Source: CAD feature listing. Evaluate the final solid. Frame: model axes, mm. Face numbers are marked on the shaded views. A direction names the side the tool comes from. Coordinates: 2 decimals unless noted, no trailing zeros. Loops run counter-clockwise (first coordinate to the right, second up) from the corner with the lowest first, then second, coordinate; pieces in that order, holes last.
Item 1: Section query B-B, the plane x = 15.5. Return the cut outline in (y, z), then the cut area to 3 significant figures.
Item 2: Reachability of the marked faces 1, 2, 3 and 4 from +Z, -Z, +X, -X, +Y, -Y: full face, straight path, thin tool, end or side. Return the list, or none.
Item 3: Section query A-A, the plane y = 5.5. Return the cut outline in (x, z), then the cut area to 3 significant figures.
Item 4: Section query C-C, the plane z = 4.5. Return the cut outline in (x, y).
Item 5: Pull-direction query (X, two-part tool) for the marked faces 5, 6, 7 and 8; classes: +X half, -X half, draft (parallel to the pull), parting line (faces both ways), or undercut.
Item 6: Section query D-D, the plane y = 2.5. Return the cut outline in (x, z), then the cut area to 3 significant figures.
Item 7: Pin query (flat end, axial travel): pin 1 Ø0.9 at (y, z) = (9, 0.5) entering from +X; pin 2 Ø1.5 at (y, z) = (6, -2) entering from -X; pin 3 Ø2.5 at (x, y) = (-8, 5.5) entering from +Z; pin 4 Ø3 at (y, z) = (5, -1.5) entering from -X. Return the tip coordinate at first contact, or that it passes through.
Item 8: Line query: probe 1 along Z at (x, y) = (-4, 10); probe 2 along X at (y, z) = (7.5, -0.25); probe 3 along Z at (x, y) = (9.5, 4.5). Output: solid intervals per line, ascending.
```python
from build123d import *

# Parameters (mm, degrees)
SKETCH1_W           = 13.5
SKETCH1_H           = 6.2
BOSS_EXTRUDE1_DEPTH = 11
SKETCH2_R           = 1.6
CUT_EXTRUDE1_DEPTH  = 30.829725108
FILLET1_R           = 1
SKETCH3_W           = 18
SKETCH3_H           = 3
CUT_EXTRUDE2_DEPTH  = 30.829725108


with BuildPart() as part:
    # Sketch1 → Boss-Extrude1 (new body)
    with BuildSketch(Plane(origin=(0, 0, 0), x_dir=(1, 0, 0), z_dir=(0, 1, 0))):
        with BuildLine():
            Line((-12, -6.25), (24.75, -6.25))
            Line((24.75, -6.25), (24.75, 6.25))
            Line((24.75, 6.25), (-12, 6.25))
            Line((-12, 6.25), (-12, 3.5))
            Line((-12, 3.5), (-2.037768387, 3.5))
            ThreePointArc((-2.037768387, 3.5), (2.018605711, 3.511086867), (4.05, 0))
            ThreePointArc((4.05, 0), (2.018605711, -3.511086867), (-2.037768387, -3.5))
            Line((-2.037768387, -3.5), (-12, -3.5))
            Line((-12, -3.5), (-12, -6.25))
        make_face()
        with Locations((15, 0)):
            Rectangle(SKETCH1_W, SKETCH1_H, mode=Mode.SUBTRACT)
    extrude(amount=BOSS_EXTRUDE1_DEPTH)

    # Sketch2 → Cut-Extrude1 (cut, through all)
    with BuildSketch(Plane.XY.offset(6.25)):
        with Locations((-8, 5.5)):
            Circle(SKETCH2_R)
    extrude(amount=-CUT_EXTRUDE1_DEPTH, mode=Mode.SUBTRACT)

    # Fillet1
    fillet1_edges = [part.edges().sort_by_distance(p)[0] for p in [
        (-12, 5.5, -6.25),
        (24.75, 5.5, -6.25),
        (24.75, 5.5, 6.25),
        (-12, 5.5, 6.25),
    ]]
    fillet(fillet1_edges, radius=FILLET1_R)

    # Sketch3 → Cut-Extrude2 (cut, through all)
    with BuildSketch(Plane.XY.offset(6.25)):
        with Locations((15.75, 9.5)):
            Rectangle(SKETCH3_W, SKETCH3_H)
    extrude(amount=-CUT_EXTRUDE2_DEPTH, mode=Mode.SUBTRACT)


solid = part.part
```
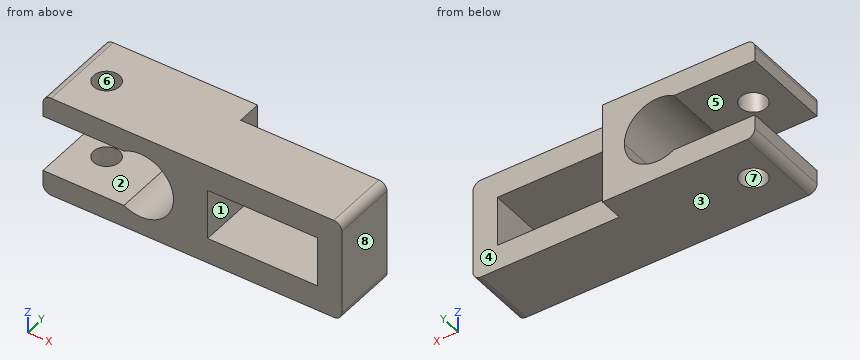
Verdict:
1. outline: (0, -6.25) - (8, -6.25) - (8, -3.1) - (0, -3.1) - close; (0, 3.1) - (8, 3.1) - (8, 6.25) - (0, 6.25) - close
1. area: 50.4 mm2
2. face 1: +Y, -Y
2. face 2: -X, +Y, -Y
2. face 3: -Z, +X, -X, +Y, -Y
2. face 4: +Z, -Z, +X, +Y
3. outline: (-12, -5.25) arc R1 ccw to (-11, -6.25) - (-9.6, -6.25) - (-9.6, -3.5) - (-12, -3.5) - close; (-12, 3.5) - (-9.6, 3.5) - (-9.6, 6.25) - (-11, 6.25) arc R1 ccw to (-12, 5.25) - close; (-6.4, -6.25) - (23.75, -6.25) arc R1 ccw to (24.75, -5.25) - (24.75, 5.25) arc R1 ccw to (23.75, 6.25) - (-6.4, 6.25) - (-6.4, 3.5) - (-2.04, 3.5) arc R4.05 cw (long way) to (-2.04, -3.5) - (-6.4, -3.5) - close; hole (8.25, -3.1) - (21.75, -3.1) - (21.75, 3.1) - (8.25, 3.1) - close
3. area: 246 mm2
4. outline: (-12, 0) - (24.75, 0) - (24.75, 8) - (6.75, 8) - (6.75, 11) - (-12, 11) - close; hole circle Ø3.2 at (-8, 5.5)
5. face 5: draft
5. face 6: undercut
5. face 7: undercut
5. face 8: +X half
6. outline: (-12, -5.25) arc R1 ccw to (-11, -6.25) - (23.75, -6.25) arc R1 ccw to (24.75, -5.25) - (24.75, 5.25) arc R1 ccw to (23.75, 6.25) - (-11, 6.25) arc R1 ccw to (-12, 5.25) - (-12, 3.5) - (-2.04, 3.5) arc R4.05 cw (long way) to (-2.04, -3.5) - (-12, -3.5) - close; hole (8.25, -3.1) - (21.75, -3.1) - (21.75, 3.1) - (8.25, 3.1) - close
6. area: 264 mm2
7. pin 1: stops at x = 6.75
7. pin 2: stops at x = 2.97
7. pin 3: passes through
7. pin 4: stops at x = 2.72
8. probe 1: z = -6.25 to -3.5, 3.5 to 6.25
8. probe 2: x = 4.04 to 8.25, 21.75 to 24.75
8. probe 3: z = -6.25 to -3.1, 3.1 to 6.25
